Geometry check sheet. Reference: the model listing, model coordinates, mm. A direction names the side the tool comes from. Give positions to 0.01 mm unless a question says otherwise; leave off trailing zeros. Loops run counter-clockwise (first coordinate to the right, second up) from the corner with the lowest first, then second, coordinate; pieces in that order, holes last. Notation, with made-up numbers: (72.25, -9.5) -> (128.25, -9.5) arc R11 cw to (128.25, -2.5) -> close; hole circle Ø3 at (-2, 81.25). An arc over 180 degrees is marked (long way). Answer as a JSON object with one key per item and string values.
Autodesk Inventor part; units mm, degrees
ref_plane "YZ Plane" through (0, 0, 0) normal (1, 0, 0) x (0, 1, 0)
ref_plane "XZ Plane" through (0, 0, 0) normal (0, 1, 0) x (-1, 0, 0)
ref_plane "XY Plane" through (0, 0, 0) normal (0, 0, 1) x (1, 0, 0)
sketch "草图1" plane through (0, 0, 0) normal (0, 0, 1) x (1, 0, 0)
  circle A0 centre (0, 0) radius 25
  dimension "d0" = 50
extrude "拉伸1" add sketch "草图1" along normal blind 5
sketch "草图2" plane through (0, 0, 5) normal (0, 0, 1) x (1, 0, 0)
  circle A0 centre (0, 0) radius 10
  line L0 (-10, 0) -> (-10, -10)
  line L1 (-10, -10) -> (10, -10)
  line L2 (10, -10) -> (10, 0)
  dimension "d3" = 20
extrude "拉伸2" cut sketch "草图2" against normal through all
sketch "草图3" plane through (0, 0, 5) normal (0, 0, 1) x (1, 0, 0)
  circle A0 centre (-17.3205, -10) radius 2.5
  circle A1 centre (17.3205, -10) radius 2.5
  circle A2 centre (0, 20) radius 2.5
  line L0 (0, 0) -> (0, 20)
  line L1 (0, 0) -> (-17.3205, -10)
  line L2 (0, 0) -> (17.3205, -10)
  dimension "d6" = 5
  dimension "d7" = 5
  dimension "d8" = 5
  dimension "d9" = 20
  dimension "d10" = 120
  dimension "d11" = 120
extrude "拉伸3" cut sketch "草图3" against normal through all
properties part number "刀夹片"
1) Section check A-A on y = -1. Record the cut outline in (x, z), plus the area to 3 significant figures.
Geometry check:
{"outline": "(-24.98, 0) -> (-10, 0) -> (-10, 5) -> (-24.98, 5) -> close; (10, 0) -> (24.98, 0) -> (24.98, 5) -> (10, 5) -> close", "area": "150 mm2"}
2) Section check D-D on x = -16. Record the cut outline in (y, z), plus the area to 3 significant figures.
Geometry check:
{"outline": "(-19.21, 0) -> (-12.12, 0) -> (-12.12, 5) -> (-19.21, 5) -> close; (-7.88, 0) -> (19.21, 0) -> (19.21, 5) -> (-7.88, 5) -> close", "area": "171 mm2"}
3) Depth check by flat-ended pin: P1, Ø3, axis at y = 10, z = 1.5, coming from the -X side; P2, Ø3, axis at y = -5, z = 1.5, coming from the +X side; P3, Ø1.5, axis at x = 5, z = 4.5, coming from the +Y side. Enter the tip coordinate at first touch or a pass-through.
Geometry check:
{"P1": "stops at x = -23.51", "P2": "stops at x = 24.75", "P3": "stops at y = 24.64"}
4) Tool access check on faces 1 (the face through (10, -5, 3)), 2 (the face through (11, 0, 0)). Record the directions out of +Z, -Z, +X, -X, +Y, -Y that give a thin tool (end or side, any length) a straight path to the whole face; none if there is none.
Geometry check:
{"face 1": "+Z, -Z", "face 2": "-Z, +X, -X, +Y, -Y"}
5) Draft check along X on faces 3 (the face through (18.47, -12.22, 2.54)), 4 (the face through (23.846, -7.509, 2.465)), 5 (the face through (11, 0, 5)). Enter one of: pulls with the +X half, pulls with the -X half, needs draft (parallel to the pull), parting line crosses it, or undercut.
Geometry check:
{"face 3": "undercut", "face 4": "parting line crosses it", "face 5": "needs draft"}
6) Section check C-C on z = 3.65. Record the cut outline in (x, y), plus the area to 3 significant figures.
Geometry check:
{"outline": "circle Ø50 at (0, 0); hole circle Ø5 at (-17.32, -10); hole (-10, -10) -> (10, -10) -> (10, 0) arc R10 ccw to (-10, 0) -> close; hole circle Ø5 at (0, 20); hole circle Ø5 at (17.32, -10)", "area": "1,550 mm2"}
7) Material ranges on line 1 along X through (y, z) = (-9, 2.15); line 2 along Y through (x, z) = (2, 4.2); line 3 along X through (y, z) = (-4.5, 4.8), recorded low to high. Write a range as from..to.
Geometry check:
{"line 1": "x = -23.32..-19.61, -15.03..-10, 10..15.03, 19.61..23.32", "line 2": "y = -24.92..-10, 9.8..18.5, 21.5..24.92", "line 3": "x = -24.59..-10, 10..24.59"}
8) Section check B-B on x = 0. Record the cut outline in (y, z).
Geometry check:
{"outline": "(-25, 0) -> (-10, 0) -> (-10, 5) -> (-25, 5) -> close; (10, 0) -> (17.5, 0) -> (17.5, 5) -> (10, 5) -> close; (22.5, 0) -> (25, 0) -> (25, 5) -> (22.5, 5) -> close"}
